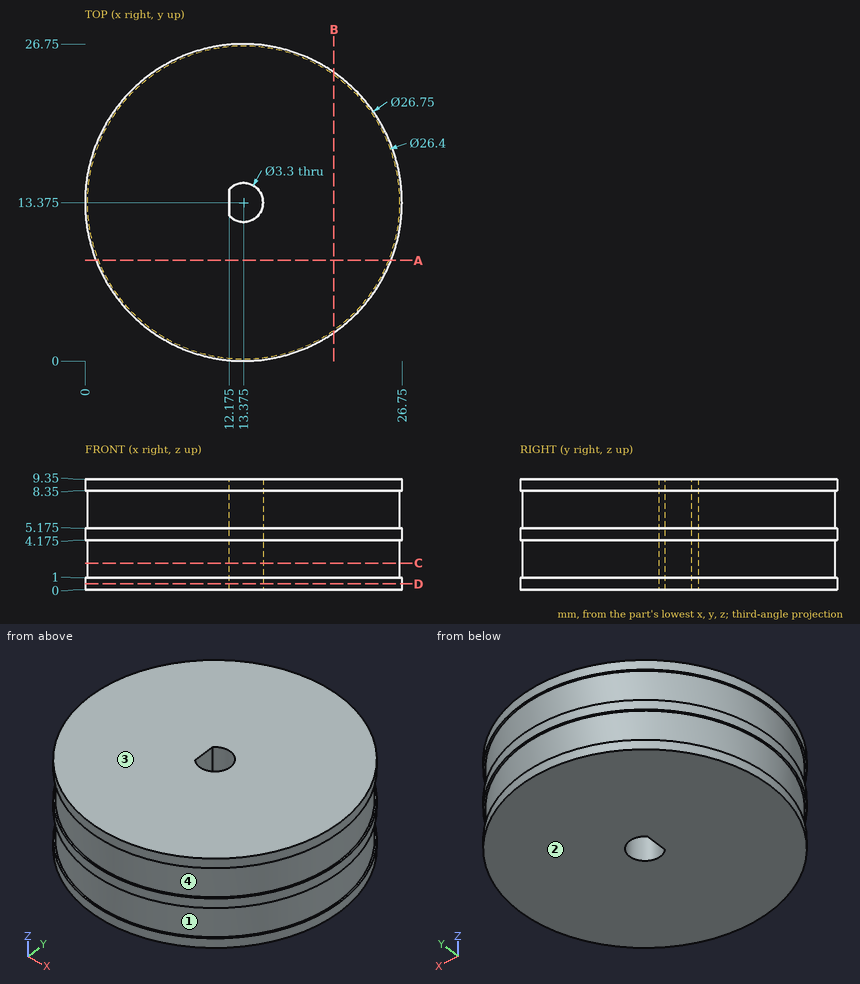
Input: dimensioned drawing with shaded views. Units: mm. Origin: part minimum x, y, z. Round coordinates to 2 decimals unless told otherwise and drop trailing zeros. Loops run counter-clockwise (first coordinate to the right, second up) from the corner with the lowest first, then second, coordinate; pieces in that order, holes last. Notation, with made-up numbers: M 52,18.25 L 99,18.25 A13 cw 99,34.25 Z; hole C 31,64 d9. An arc over 180 degrees is marked long. Answer in a Markdown table with one row per item. Add a question column.
1. Section A-A (y = 8.5). Output: boundary loops of the cut face in (x, z) (3 decimals).
2. Section C-C (z = 2.25). Output: boundary loops of the cut face in (x, y) (3 decimals), and give its area (3 significant figures).
3. Mould query, pull axis Z, two halves, no side actions, for the marked faces 1, 2, 3 and 4. Classes: released by +Z, released by -Z, zero draft, split by the parting line, or undercut.
4. Section B-B (x = 21). Output: boundary loops of the cut face in (y, z) (3 decimals).
5. Ray query, probe 1 along Y at (x, z) = (13.5, 3.25); probe 2 along X at (y, z) = (13.25, 3) (3 decimals); probe 3 along X at (y, z) = (14.5, 3.25) (3 decimals). Return the intervals inside material, ascending.
6. Contact query for flat-ended pins moving along their axis: pin 1 (4 mm diameter, centred on x = 7, z = 4.5, fed in from +Y); pin 2 (3 mm diameter, centred on y = 9.5, z = 1, fed in from +X); pin 3 (1.5 mm diameter, centred on x = 16, z = 1, fed in from +Y). Output: stop coordinate, or through.
7. Section D-D (z = 0.5). Output: boundary loops of the cut face in (x, y) (3 decimals).
Values follow:
| question | item | result |
|---|---|---|
| 1 | outline | M 0.92,0 L 25.83,0 L 25.83,1 L 25.642,1 L 25.642,4.175 L 25.83,4.175 L 25.83,5.175 L 25.642,5.175 L 25.642,8.35 L 25.83,8.35 L 25.83,9.35 L 0.92,9.35 L 0.92,8.35 L 1.108,8.35 L 1.108,5.175 L 0.92,5.175 L 0.92,4.175 L 1.108,4.175 L 1.108,1 L 0.92,1 Z |
| 2 | outline | C 13.375,13.375 d26.4; hole M 12.175,12.243 A1.65 ccw long 12.175,14.507 Z |
| 2 | area | 540 mm^2 |
| 3 | face 1 | undercut |
| 3 | face 2 | released by -Z |
| 3 | face 3 | released by +Z |
| 3 | face 4 | undercut |
| 4 | outline | M 2.386,0 L 24.364,0 L 24.364,1 L 24.15,1 L 24.15,4.175 L 24.364,4.175 L 24.364,5.175 L 24.15,5.175 L 24.15,8.35 L 24.364,8.35 L 24.364,9.35 L 2.386,9.35 L 2.386,8.35 L 2.6,8.35 L 2.6,5.175 L 2.386,5.175 L 2.386,4.175 L 2.6,4.175 L 2.6,1 L 2.386,1 Z |
| 5 | probe 1 | 0.18 to 11.73, 15.02 to 26.57 |
| 5 | probe 2 | 0.176 to 12.175, 15.02 to 26.574 |
| 5 | probe 3 | 0.223 to 12.175, 14.582 to 26.527 |
| 6 | pin 1 | y = 26.01 |
| 6 | pin 2 | x = 26.54 |
| 6 | pin 3 | y = 26.62 |
| 7 | outline | C 13.375,13.375 d26.75; hole M 12.175,12.243 A1.65 ccw long 12.175,14.507 Z |
